```python
from build123d import *

# Parameters (mm, degrees)
SKICA4_R                 = 23.5
P_IDAT_VYSUNUT_M1_DEPTH  = 3
SKICA6_R                 = 16.78
ODEBRAT_VYSUNUT_M2_DEPTH = 3
SKICA7_W                 = 3
SKICA7_H                 = 6.382195619
SKICA7_W_2               = 6.382195619
SKICA7_H_2               = 3
ODEBRAT_VYSUNUT_M3_DEPTH = 3


with BuildPart() as part:
    # Skica4 → Přidat vysunutím1 (new body)
    with BuildSketch(Plane(origin=(0, 0, 0), x_dir=(1, 0, 0), z_dir=(0, 1, 0))):
        with Locations(Location((0, 0, 0), (0, 0, 270))):
            Circle(SKICA4_R)
    extrude(amount=P_IDAT_VYSUNUT_M1_DEPTH)

    # Skica6 → Odebrat vysunutím2 (cut)
    with BuildSketch(Plane.XZ):
        with Locations(Location((0, 0, 0), (0, 0, 270))):
            Circle(SKICA6_R)
    extrude(amount=-ODEBRAT_VYSUNUT_M2_DEPTH, mode=Mode.SUBTRACT)

    # Skica7 → Odebrat vysunutím3 (cut)
    with BuildSketch(Plane(origin=(0, 3, 0), x_dir=(1, 0, 0), z_dir=(0, 1, 0))):
        with Locations((0, -22.69109781)):
            Rectangle(SKICA7_W, SKICA7_H)
        with Locations((22.69109781, 0)):
            Rectangle(SKICA7_W_2, SKICA7_H_2)
        with Locations((-22.69109781, 0)):
            Rectangle(SKICA7_W_2, SKICA7_H_2)
        with Locations((0, 22.69109781)):
            Rectangle(SKICA7_W, SKICA7_H)
    extrude(amount=-ODEBRAT_VYSUNUT_M3_DEPTH, mode=Mode.SUBTRACT)


solid = part.part
```
Read the model definition and answer for the solid it produces. Units are mm, in the model's axes. A direction names the side the tool comes from. Coordinates: 2 decimals unless noted, no trailing zeros. Loops run counter-clockwise (first coordinate to the right, second up) from the corner with the lowest first, then second, coordinate; pieces in that order, holes last.
(1) The part is cut by section B-B (x = 0). Determine the outline of the cut face in (y, z), and give its area (3 significant figures).
Solution:
outline: (0, -19.5) - (3, -19.5) - (3, -16.78) - (0, -16.78) - close; (0, 16.78) - (3, 16.78) - (3, 19.5) - (0, 19.5) - close
area: 16.3 mm2
(2) A tool of negligible diameter and unlimited length cuts with its end or side. For faces 4 (the face through (-1.5, 2, -21)), 5 (the face through (-1.5, 2, 22)), 6 (the face through (-19.5, 2, 0)), 7 (the face through (21, 2, -1.5)), from which of +Z, -Z, +X, -X, +Y, -Y can it reach the whole face along a straight path? Write none if from no direction.
Solution:
face 4: -Z, +Y, -Y
face 5: +Z, +Y, -Y
face 6: -X, +Y, -Y
face 7: +X, +Y, -Y
(3) The part is cut by section C-C (y = 2.15). Determine the outline of the cut face in (x, z), and give its area (3 significant figures).
Solution:
outline: (-23.45, -1.5) arc R23.5 ccw to (-1.5, -23.45) - (-1.5, -19.5) - (1.5, -19.5) - (1.5, -23.45) arc R23.5 ccw to (23.45, -1.5) - (19.5, -1.5) - (19.5, 1.5) - (23.45, 1.5) arc R23.5 ccw to (1.5, 23.45) - (1.5, 19.5) - (-1.5, 19.5) - (-1.5, 23.45) arc R23.5 ccw to (-23.45, 1.5) - (-19.5, 1.5) - (-19.5, -1.5) - close; hole circle Ø33.56 at (0, 0)
area: 803 mm2
(4) Consider line 1 along X through (y, z) = (1.4, 0); line 2 along X through (y, z) = (1.65, -8); line 3 along Z through (x, y) = (-8.5, 1.65). Determine where each line is inside the solid, lowest interval first.
Solution:
line 1: x = -19.5 to -16.78, 16.78 to 19.5
line 2: x = -22.1 to -14.75, 14.75 to 22.1
line 3: z = -21.91 to -14.47, 14.47 to 21.91
(5) Flat-ended cylindrical pins translate along their axes: pin 1 Ø1.5 at (y, z) = (2, 0) entering from -X; pin 2 Ø1.5 at (x, y) = (0.5, 1.5) entering from -Z; pin 3 Ø1.5 at (x, y) = (-21, 2) entering from -Z. Find the tip coordinate at first contact, or state that the pin passes through.
Solution:
pin 1: stops at x = -19.5
pin 2: stops at z = -19.5
pin 3: stops at z = -11.92
(6) The mould has two halves that part along X. Classify faces 1 (the face through (1.5, 2, -21)), 2 (the face through (-16, 3, -7)), 3 (the face through (-16.45, 1.48, -16.78)): released by +X, released by -X, zero draft, split by the parting line, or undercut.
Solution:
face 1: undercut
face 2: zero draft
face 3: released by -X
(7) The part is cut by section A-A (z = 0). Determine the outline of the cut face in (x, y).
Solution:
outline: (-19.5, 0) - (-16.78, 0) - (-16.78, 3) - (-19.5, 3) - close; (16.78, 0) - (19.5, 0) - (19.5, 3) - (16.78, 3) - close
